Part print with two shaded views. Sizes in mm from the minimum x, y, z corner. A direction names the side the tool comes from. Round coordinates to 2 decimals unless told otherwise and drop trailing zeros. Loops run counter-clockwise (first coordinate to the right, second up) from the corner with the lowest first, then second, coordinate; pieces in that order, holes last. Notation, with made-up numbers: (-37.5, 17) -> (-7.5, 17) arc R26 ccw to (-7.5, 47) -> close; hole circle Ø2 at (5, 11). An arc over 180 degrees is marked (long way). Use a Markdown table: item, result. Add a question column.
Item 1: Cut at D-D, the plane y = 7. List the corners of the cut face in (x, z), plus the area to 3 significant figures.
Item 2: Cut at C-C, the plane z = 2.45. List the corners of the cut face in (x, y).
Item 3: Cut at A-A, the plane x = 25. List the corners of the cut face in (y, z), plus the area to 3 significant figures.
Item 4: Which spindle directions (+Z, -Z, +X, -X, +Y, -Y) get a long thin tool onto all of the face, cutting with end or side? Do the marked faces 1, 2 and 3. Say none if no direction does.
Item 5: Probe line 1 (Y direction, x = 25, z = 1.4); line 2 (Y direction, x = 9, z = 4.5); line 3 (Y direction, x = 25.5, z = 4.85). List the from-to ranges inside material, lowest first. Write a range as [from, to].
Item 6: Flat gauge pins, fed straight in: pin 1 (2 mm diameter, centred on x = 24.5, y = 38, fed in from +Z); pin 2 (1.5 mm diameter, centred on y = 24.5, z = 4.5, fed in from +X); pin 3 (2 mm diameter, centred on x = 8, z = 4.5, fed in from -Y); pin 4 (3 mm diameter, centred on y = 10.5, z = 2, fed in from -X). Where does each tip first touch, or does it go through?
Item 7: Cut at B-B, the plane y = 37. List the corners of the cut face in (x, z), plus the area to 3 significant figures.
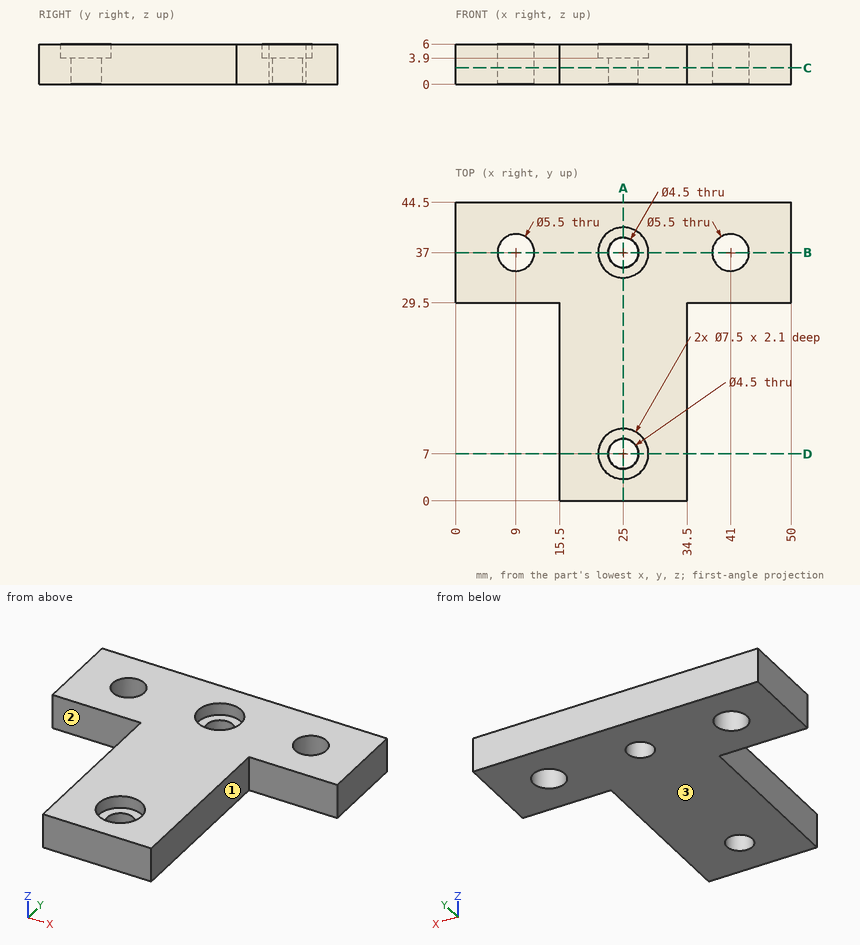
A:
| question | item | result |
|---|---|---|
| 1 | outline | (15.5, 0) -> (22.75, 0) -> (22.75, 3.9) -> (21.25, 3.9) -> (21.25, 6) -> (15.5, 6) -> close; (27.25, 0) -> (34.5, 0) -> (34.5, 6) -> (28.75, 6) -> (28.75, 3.9) -> (27.25, 3.9) -> close |
| 1 | area | 80.7 mm^2 |
| 2 | outline | (0, 29.5) -> (15.5, 29.5) -> (15.5, 0) -> (34.5, 0) -> (34.5, 29.5) -> (50, 29.5) -> (50, 44.5) -> (0, 44.5) -> close; hole circle Ø5.5 at (9, 37); hole circle Ø4.5 at (25, 7); hole circle Ø4.5 at (25, 37); hole circle Ø5.5 at (41, 37) |
| 3 | outline | (0, 0) -> (4.75, 0) -> (4.75, 3.9) -> (3.25, 3.9) -> (3.25, 6) -> (0, 6) -> close; (9.25, 0) -> (34.75, 0) -> (34.75, 3.9) -> (33.25, 3.9) -> (33.25, 6) -> (10.75, 6) -> (10.75, 3.9) -> (9.25, 3.9) -> close; (39.25, 0) -> (44.5, 0) -> (44.5, 6) -> (40.75, 6) -> (40.75, 3.9) -> (39.25, 3.9) -> close |
| 3 | area | 200 mm^2 |
| 4 | face 1 | +Z, -Z, +X, -Y |
| 4 | face 2 | +Z, -Z, -X, -Y |
| 4 | face 3 | -Z, +X, -X, +Y, -Y |
| 5 | line 1 | y = [0, 4.75], [9.25, 34.75], [39.25, 44.5] |
| 5 | line 2 | y = [29.5, 34.25], [39.75, 44.5] |
| 5 | line 3 | y = [0, 3.28], [10.72, 33.28], [40.72, 44.5] |
| 6 | pin 1 | passes through |
| 6 | pin 2 | stops at x = 34.5 |
| 6 | pin 3 | stops at y = 29.5 |
| 6 | pin 4 | stops at x = 15.5 |
| 7 | outline | (0, 0) -> (6.25, 0) -> (6.25, 6) -> (0, 6) -> close; (11.75, 0) -> (22.75, 0) -> (22.75, 3.9) -> (21.25, 3.9) -> (21.25, 6) -> (11.75, 6) -> close; (27.25, 0) -> (38.25, 0) -> (38.25, 6) -> (28.75, 6) -> (28.75, 3.9) -> (27.25, 3.9) -> close; (43.75, 0) -> (50, 0) -> (50, 6) -> (43.75, 6) -> close |
| 7 | area | 201 mm^2 |
